```python
from build123d import *

# Parameters (mm, degrees)
SKETCH_1_W      = 21.5
SKETCH_1_H      = 11.8
EXTRUDE_1_DEPTH = 22.7
EXTRUDE_2_DEPTH = 3
SKETCH_3_R      = 2
SKETCH_3_R_2    = 0.8
EXTRUDE_3_DEPTH = 7.4
SKETCH_6_R      = 4
EXTRUDE_4_DEPTH = 3


with BuildPart() as part:
    # 草图1 → 凸台-拉伸1 (new body)
    with BuildSketch(Plane(origin=(0, 0, 0), x_dir=(1, 0, 0), z_dir=(0, 1, 0))):
        with Locations((10.75, -5.9)):
            Rectangle(SKETCH_1_W, SKETCH_1_H)
    extrude(amount=EXTRUDE_1_DEPTH)

    # 草图2 → 凸台-拉伸2 (add)
    with BuildSketch(Plane(origin=(0, 16.1, 0), x_dir=(1, 0, 0), z_dir=(0, 1, 0))):
        with BuildLine():
            Line((-5.35, -11.8), (0, -11.8))
            Line((0, -11.8), (0, 0))
            Line((0, 0), (-5.35, 0))
            Line((-5.35, 0), (-5.35, -5.4))
            Line((-5.35, -5.4), (-4.016025404, -5.4))
            ThreePointArc((-4.016025404, -5.4), (-2.15, -5.9), (-4.016025404, -6.4))
            Line((-4.016025404, -6.4), (-5.35, -6.4))
            Line((-5.35, -6.4), (-5.35, -11.8))
        make_face()
        with BuildLine():
            Line((26.85, 0), (21.5, 0))
            Line((21.5, 0), (21.5, -11.8))
            Line((21.5, -11.8), (26.85, -11.8))
            Line((26.85, -11.8), (26.85, -6.4))
            Line((26.85, -6.4), (25.516025404, -6.4))
            ThreePointArc((25.516025404, -6.4), (23.65, -5.9), (25.516025404, -5.4))
            Line((25.516025404, -5.4), (26.85, -5.4))
            Line((26.85, -5.4), (26.85, 0))
        make_face()
    extrude(amount=EXTRUDE_2_DEPTH)

    # 草图3 → 凸台-拉伸3 (add)
    with BuildSketch(Plane(origin=(0, 22.7, 0), x_dir=(1, 0, 0), z_dir=(0, 1, 0))):
        with Locations(Location((15.65, -5.9, 0), (0, 0, 270))):
            Circle(SKETCH_3_R)
        with Locations(Location((15.65, -5.9, 0), (0, 0, 270))):
            Circle(SKETCH_3_R_2, mode=Mode.SUBTRACT)
    extrude(amount=EXTRUDE_3_DEPTH)

    # 草图6 → 凸台-拉伸4 (add)
    with BuildSketch(Plane(origin=(0, 22.7, 0), x_dir=(1, 0, 0), z_dir=(0, 1, 0))):
        with Locations(Location((15.65, -5.9, 0), (0, 0, 270))):
            Circle(SKETCH_6_R)
    extrude(amount=EXTRUDE_4_DEPTH)


solid = part.part
```
Part model, mm, in its own coordinate system. A direction names the side the tool comes from. Coordinates: 2 decimals unless noted, no trailing zeros. Order: outer loops, then holes, each group sorted by start corner. A loop starts at its lowest first (then second) coordinate and runs counter-clockwise, first axis right, second up. Notation, with made-up numbers: (4.5, 73.5) - (28.5, 73.5) arc R21 ccw to (28.5, 77.5) - close; hole circle Ø9 at (-5, 10). An arc over 180 degrees is marked (long way). Return JSON: item names as keys, results as strings. Group by question number.
Item 1: Pin check, flat tips, straight feed: pin 1 (1.1 mm diameter, centred on y = 21, z = 6, fed in from +X); pin 2 (1.2 mm diameter, centred on x = -3.15, z = 5.9, fed in from -Y); pin 3 (4 mm diameter, centred on y = 22, z = 7.5, fed in from -X); pin 4 (2.5 mm diameter, centred on x = -1.5, z = 6, fed in from +Y). Stop position of each tip, or through.
Item 2: Drill centre lines: probe 1 along Z at (x, y) = (15.65, 27.7); probe 2 along X at (y, z) = (21.5, 8); probe 3 along Y at (x, z) = (2, 4). Where is each one in solid material? Low to high. Write a range as from..to.
Item 3: Cut at C-C (x = 15.65). List the corners of the cut face in (y, z), plus the area to 3 significant figures.
Item 4: Pull direction Z, two halves, no side cores. Call faces 4 (the face through (11, 11, 11.8)), 5 (the face through (14.433, 27.869, 4.313)), 6 (the face through (26.85, 18, 9)), 7 (the face through (16.325, 27.869, 6.33)): pulls with the +Z half, pulls with the -Z half, needs draft (parallel to the pull), parting line crosses it, or undercut.
Item 5: Cut at B-B (z = 11). List the corners of the cut face in (x, y).
Item 6: Cut at A-A (x = 24.65). List the corners of the cut face in (y, z), plus the area to 3 significant figures.
Item 7: Cut at D-D (y = 3). List the corners of the cut face in (x, z).
Item 8: Which spindle directions (+Z, -Z, +X, -X, +Y, -Y) get a long thin tool onto all of the face, cutting with end or side? Do faces 1 (the face through (-5, 18, 6.4)), 2 (the face through (23.5, 16.1, 5.8)), 3 (the face through (0, 8, 6)). Say none if no direction does.
Check values:
{
 "1": {"pin 1": "stops at x = 21.5", "pin 2": "passes through", "pin 3": "stops at x = 0", "pin 4": "stops at y = 19.1"},
 "2": {"probe 1": "z = 3.9..5.1, 6.7..7.9", "probe 2": "x = 0..21.5", "probe 3": "y = 0..22.7"},
 "3": {"outline": "(0, 0) - (22.7, 0) - (22.7, 1.9) - (25.7, 1.9) - (25.7, 3.9) - (30.1, 3.9) - (30.1, 5.1) - (25.7, 5.1) - (25.7, 6.7) - (30.1, 6.7) - (30.1, 7.9) - (25.7, 7.9) - (25.7, 9.9) - (22.7, 9.9) - (22.7, 11.8) - (0, 11.8) - close", "area": "302 mm2"},
 "4": {"face 4": "pulls with the +Z half", "face 5": "parting line crosses it", "face 6": "needs draft", "face 7": "undercut"},
 "5": {"outline": "(-5.35, 16.1) - (0, 16.1) - (0, 0) - (21.5, 0) - (21.5, 16.1) - (26.85, 16.1) - (26.85, 19.1) - (21.5, 19.1) - (21.5, 22.7) - (0, 22.7) - (0, 19.1) - (-5.35, 19.1) - close"},
 "6": {"outline": "(16.1, 0) - (19.1, 0) - (19.1, 4.9) - (16.1, 4.9) - close; (16.1, 6.9) - (19.1, 6.9) - (19.1, 11.8) - (16.1, 11.8) - close", "area": "29.4 mm2"},
 "7": {"outline": "(0, 0) - (21.5, 0) - (21.5, 11.8) - (0, 11.8) - close"},
 "8": {"face 1": "-X, +Y, -Y", "face 2": "+Z, -Z, +X, -Y", "face 3": "+Z, -Z, -X, -Y"}
}
